Read the model definition and answer for the solid it produces. Units are mm, in the model's axes. Round coordinates to 2 decimals unless told otherwise and drop trailing zeros. Order: outer loops, then holes, each group sorted by start corner. A loop starts at its lowest first (then second) coordinate and runs counter-clockwise, first axis right, second up. Notation, with made-up numbers: (65, 2) - (102, 2) arc R21 ccw to (102, 8) - close; hole circle Ø2 at (18.5, 33.5). An arc over 180 degrees is marked (long way). Put each result on its own line as item: value. Start each with the question number.
Q1. Each of these flat-tipped pins is pushed along its axis until it touches: pin 1 Ø0.5 at (x, z) = (22, -2.5) entering from -Y; pin 2 Ø1 at (x, z) = (12.5, -2) entering from +Y. Where does it stop, or does it pass through?
Q2. Find the intervals of material crossed by line 1 along Y through (x, z) = (20.5, -0.55); line 2 along X through (y, z) = (11.75, -1.35); line 3 along X through (y, z) = (4, -0.35), in increasing order. Write a range as from..to.
Q3. Section A-A on z = -0.9 is taken. Give the vertices of the cut face in (x, y), then the cut area to 3 significant figures.
from build123d import *

# Parameters (mm, degrees)
F1_DEPTH = 3
F2_R     = 1.49999
F5_DEPTH = 1


# Not quite as in the source:
# - a fillet or chamfer is up to 0.001 mm smaller than in the source, because OpenCascade refuses the exact size
# - a feature names something its author has since deleted; it is built from what else it names


with BuildPart() as f1:
    # F0 (on Top) → F1 (new body)
    with BuildSketch(Plane.XY):
        with BuildLine():
            ThreePointArc((7.7126204308, 17.4904861667), (5.8623387123, 16.6961416403), (4.9310753592, 14.9108477622))
            Line((4.9310753592, 14.9108477622), (3.2946010031, 3.1761362209))
            ThreePointArc((3.2946010031, 3.1761362209), (4.002766576, 0.7923969722), (6.265847815, -0.2382215753))
            Line((6.265847815, -0.2382215753), (42.381050937, -0.2382215753))
            ThreePointArc((42.381050937, -0.2382215753), (43.9792635765, 0.2229368859), (45.0861233616, 1.4646341854))
            Line((45.0861233616, 1.4646341854), (51.9699000588, 15.820103651))
            ThreePointArc((51.9699000588, 15.820103651), (51.7518427103, 18.7949713512), (49.0751258939, 20.1112440911))
            Line((49.0751258939, 20.1112440911), (7.7126204308, 17.4904861667))
        make_face()
        with BuildLine():
            Line((39.8630322028, 3.7617784247), (10.8623798602, 3.7617784247))
            ThreePointArc((10.8623798602, 3.7617784247), (8.5992986212, 4.7923969722), (7.8911330484, 7.1761362209))
            Line((7.8911330484, 7.1761362209), (8.4418632915, 11.125272678))
            ThreePointArc((8.4418632915, 11.125272678), (9.3731266446, 12.9105665561), (11.2234083631, 13.7049110825))
            Line((11.2234083631, 13.7049110825), (42.5178482436, 15.6877491719))
            ThreePointArc((42.5178482436, 15.6877491719), (45.19456506, 14.3714764321), (45.4126224085, 11.3966087319))
            Line((45.4126224085, 11.3966087319), (42.5681046274, 5.4646341854))
            ThreePointArc((42.5681046274, 5.4646341854), (41.4612448422, 4.2229368859), (39.8630322028, 3.7617784247))
        make_face(mode=Mode.SUBTRACT)
    extrude(amount=-F1_DEPTH)

    # F2 (radius 1.5 in the source; OpenCascade refuses exactly that, so slightly less here)
    f2_edges = [f1.edges().sort_by_distance(p)[0] for p in [
        (24.323449, -0.238222, 0),
        (48.528012, 8.642369, 0),
        (28.393873, 18.800865, 0),
        (4.112838, 9.043492, 0),
        (25.362706, 3.761778, 0),
        (8.166498, 9.150704, 0),
        (43.990364, 8.430621, 0),
        (26.870628, 14.69633, 0),
        (8.166498, 9.150704, -3),
        (25.362706, 3.761778, -3),
        (26.870628, 14.69633, -3),
        (43.990364, 8.430621, -3),
    ]]
    fillet(f2_edges, radius=F2_R)

    # F4 (on offset) → F5 (cut)
    with BuildSketch(Plane(origin=(0, 0, -3), x_dir=(1, 0, 0), z_dir=(0, 0, -1))):
        with BuildLine():
            Line((3.2946010031, -3.1761362209), (4.9310753592, -14.9108477622))
            ThreePointArc((4.9310753592, -14.9108477622), (5.8623387123, -16.6961416403), (7.7126204308, -17.4904861667))
            Line((7.7126204308, -17.4904861667), (49.0751258939, -20.1112440911))
            ThreePointArc((49.0751258939, -20.1112440911), (51.7518427103, -18.7949713512), (51.9699000588, -15.820103651))
            Line((51.9699000588, -15.820103651), (45.0861233616, -1.4646341854))
            ThreePointArc((45.0861233616, -1.4646341854), (43.9792635765, -0.2229368859), (42.381050937, 0.2382215753))
            Line((42.381050937, 0.2382215753), (6.265847815, 0.2382215753))
            ThreePointArc((6.265847815, 0.2382215753), (4.002766576, -0.7923969722), (3.2946010031, -3.1761362209))
        make_face()
        with BuildLine():
            ThreePointArc((50.6173638465, -16.4686757707), (50.5083351723, -17.9561096208), (49.1699767641, -18.6142459907))
            Line((49.1699767641, -18.6142459907), (7.8074713009, -15.9934880663))
            ThreePointArc((7.8074713009, -15.9934880663), (6.8823304417, -15.5963158031), (6.4166987651, -14.7036688641))
            Line((6.4166987651, -14.7036688641), (4.7802244091, -2.9689573228))
            ThreePointArc((4.7802244091, -2.9689573228), (5.1343071955, -1.7770876984), (6.265847815, -1.2617784247))
            Line((6.265847815, -1.2617784247), (42.381050937, -1.2617784247))
            ThreePointArc((42.381050937, -1.2617784247), (43.1801572567, -1.4923576553), (43.7335871493, -2.113206305))
            Line((43.7335871493, -2.113206305), (50.6173638465, -16.4686757707))
        make_face(mode=Mode.SUBTRACT)
    extrude(amount=-F5_DEPTH, mode=Mode.SUBTRACT)


solid = f1.part
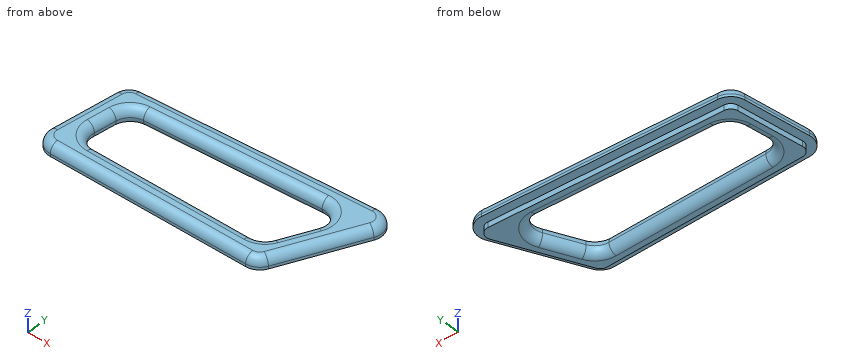
Findings:
1. pin 1: y = 1.26
1. pin 2: y = 17.83
2. line 1: 0.1..3.42, 14.63..17.96
2. line 2: 4.5..8.59, 45.56..50.01
2. line 3: 3.95..8.65, 42.07..45.71
3. outline: (3.42, 3.16) arc R2.87 ccw to (6.27, -0.11) - (42.38, -0.11) arc R2.87 ccw to (44.97, 1.52) - (51.86, 15.87) arc R2.87 ccw to (49.08, 19.99) - (7.72, 17.37) arc R2.87 ccw to (5.06, 14.89) - close; hole (7.77, 7.19) arc R3.13 ccw to (10.86, 3.64) - (39.86, 3.64) arc R3.13 ccw to (42.68, 5.41) - (45.53, 11.34) arc R3.13 ccw to (42.51, 15.81) - (11.22, 13.83) arc R3.13 ccw to (8.32, 11.14) - close
3. area: 429 mm2
